Here's the drawing with two shaded views (mm, measured from the low corner). I have some questions. A direction names the side the tool comes from. Coordinates: 2 decimals unless noted, no trailing zeros. Write each loop counter-clockwise with the first axis right and the second up, starting at its lowest first coordinate (ties: lowest second). Pieces come first, ordered by that corner, then holes. Notation, with made-up numbers: (-34, -18) -> (-9, -18) arc R28 cw to (-9, 16) -> close; hole circle Ø2 at (64, 23.25). An arc over 180 degrees is marked (long way). Put each result on its own line as item: value. Start each with the question number.
Item 1: I want a section at A-A, the plane z = 66. List the corners of the cut face in (x, y) for me, then the cut area to 3 significant figures.
Item 2: On a 3-axis mill with a long thin cutter (end or side, diameter ignored), from which of +Z, -Z, +X, -X, +Y, -Y can I reach the whole of each face in a straight line? I mean the marked faces 1, 2 and 3. Say none if no direction works.
Item 3: I want a section at C-C, the plane x = 13. List the corners of the cut face in (y, z) for me, then the cut area to 3 significant figures.
Item 4: I want a section at B-B, the plane y = 14.5. List the corners of the cut face in (x, z) for me, then the cut area to 3 significant figures.
Item 5: I need wall thicknesses on line 1 (X direction, y = 28, z = 72.5); line 2 (Y direction, x = 76, z = 54); line 3 (Y direction, x = 79, z = 61). Which ranges of each line are inside material? Lowest first, please. Write a range as [from, to].
Item 6: If we mould it in two halves opening along X, with no side actions, what happens to the marked faces 4, 5, 6 and 7? For each: released by +X, released by -X, zero draft, split by the parting line, or undercut.
Item 7: For pin 1 (15 mm diameter, centred on x = 44.5, y = 22, fed in from +Z); pin 2 (15 mm diameter, centred on x = 67, z = 50.5, fed in from -Y), each with a flat end and sliding along its axis, tell me the tip position at first contact or that it passes through.
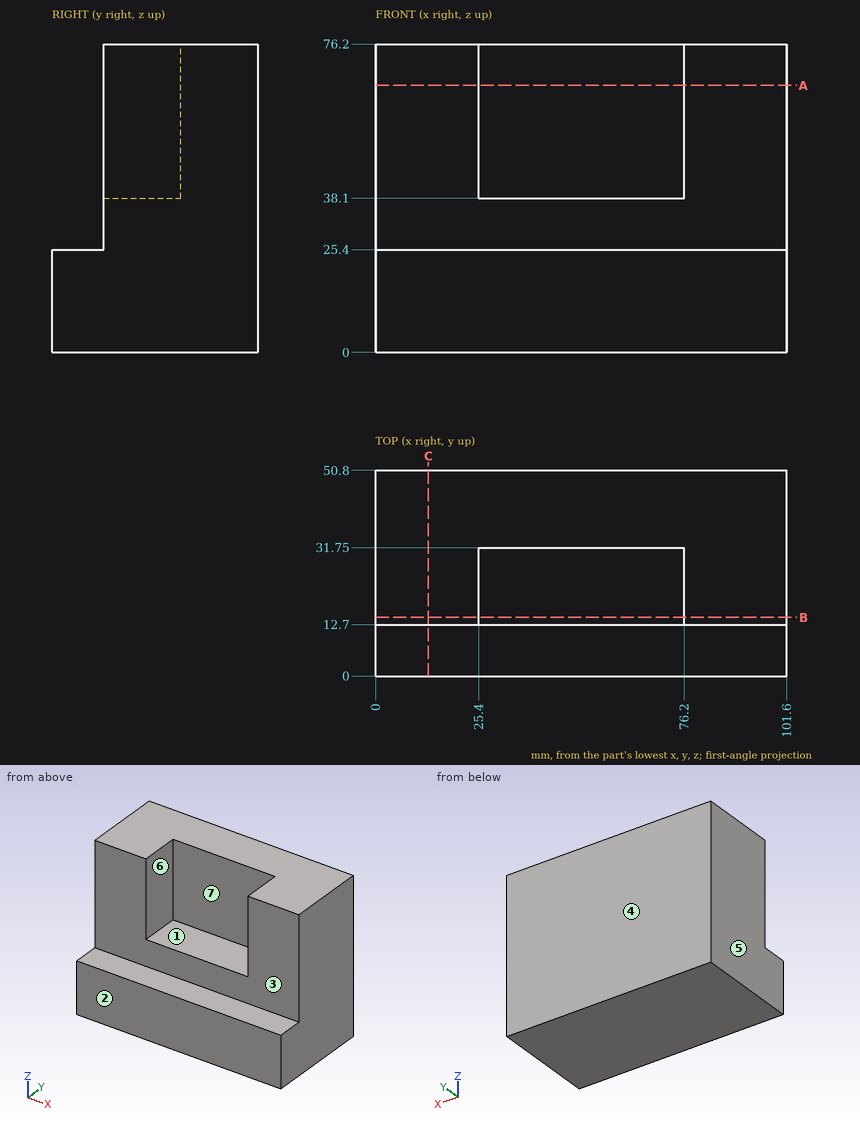
Calculated:
1. outline: (0, 12.7) -> (25.4, 12.7) -> (25.4, 31.75) -> (76.2, 31.75) -> (76.2, 12.7) -> (101.6, 12.7) -> (101.6, 50.8) -> (0, 50.8) -> close
1. area: 2,900 mm2
2. face 1: +Z, -Y
2. face 2: +Z, -Z, +X, -X, -Y
2. face 3: +Z, +X, -X, -Y
3. outline: (0, 0) -> (50.8, 0) -> (50.8, 76.2) -> (12.7, 76.2) -> (12.7, 25.4) -> (0, 25.4) -> close
3. area: 3,230 mm2
4. outline: (0, 0) -> (101.6, 0) -> (101.6, 76.2) -> (76.2, 76.2) -> (76.2, 38.1) -> (25.4, 38.1) -> (25.4, 76.2) -> (0, 76.2) -> close
4. area: 5,810 mm2
5. line 1: x = [0, 25.4], [76.2, 101.6]
5. line 2: y = [31.75, 50.8]
5. line 3: y = [12.7, 50.8]
6. face 4: zero draft
6. face 5: released by -X
6. face 6: undercut
6. face 7: undercut
7. pin 1: stops at z = 38.1
7. pin 2: stops at y = 31.75
